Check sheet for the modelled part. Datum: model origin and axes. Units: mm. Give positions to 0.01 mm unless a question says otherwise; leave off trailing zeros. Loops run counter-clockwise (first coordinate to the right, second up) from the corner with the lowest first, then second, coordinate; pieces in that order, holes last.
```python
from build123d import *

# Parameters (mm, degrees)
SKETCH1_R           = 1.5
BOSS_EXTRUDE1_DEPTH = 3


with BuildPart() as part:
    # Sketch1 → Boss-Extrude1 (new body)
    with BuildSketch(Plane.XY):
        with BuildLine():
            Line((15.435057436, 20.921377099), (-0.10870117, 20.838196592))
            ThreePointArc((-0.10870117, 20.838196592), (-2.225289061, 19.948177695), (-3.092604315, 17.822185647))
            Line((-3.092604315, 17.822185647), (-2.998956565, 0.322436217))
            ThreePointArc((-2.998956565, 0.322436217), (-2.108937668, -1.794151674), (0.01705438, -2.661466928))
            Line((0.01705438, -2.661466928), (15.560812986, -2.578286421))
            ThreePointArc((15.560812986, -2.578286421), (17.766430895, -3.332819275), (19.891460268, -2.374528948))
            Line((19.891460268, -2.374528948), (30.659457178, -1.580311749))
            ThreePointArc((30.659457178, -1.580311749), (32.311987692, -0.938952483), (33.323696389, 0.516603879))
            ThreePointArc((33.323696389, 0.516603879), (33.38449749, 2.903690209), (32.146093551, 4.945315446))
            Line((32.146093551, 4.945315446), (32.099909063, 13.575709212))
            ThreePointArc((32.099909063, 13.575709212), (33.31639169, 15.630471471), (33.230046407, 18.016770366))
            ThreePointArc((33.230046407, 18.016770366), (32.202817639, 19.461415605), (30.543517656, 20.085052019))
            Line((30.543517656, 20.085052019), (19.767637393, 20.763979817))
            ThreePointArc((19.767637393, 20.763979817), (17.632473675, 21.699472247), (15.435057436, 20.921377099))
        make_face()
        with Locations((29.560164558, 17.392133017)):
            Circle(SKETCH1_R, mode=Mode.SUBTRACT)
        with Locations((29.65, 0.604781235)):
            Circle(SKETCH1_R, mode=Mode.SUBTRACT)
        with Locations((-0.101138608, 0.73794926)):
            Circle(SKETCH1_R, mode=Mode.SUBTRACT)
        with Locations((-0.190505318, 17.437710144)):
            Circle(SKETCH1_R, mode=Mode.SUBTRACT)
        Polygon((2.641027261, 11.552778262), (2.667248631, 6.652848422), (4.067228585, 6.660340242), (4.089168915, 2.560398947), (9.689088733, 2.590366227), (9.704072373, -0.209593682), (21.903897689, -0.144307821), (21.888914049, 2.655652087), (27.388835298, 2.685084237), (27.321944048, 15.184905259), (24.621982708, 15.170456748), (24.605393678, 18.270412362), (9.605608452, 18.190142862), (9.622197482, 15.090187248), (4.022277665, 15.060219968), (4.041007215, 11.560270082), align=None, mode=Mode.SUBTRACT)
    extrude(amount=BOSS_EXTRUDE1_DEPTH)


solid = part.part
```
(1) Release check for a two-part mould opening along Y. For faces 1 (the face through (32.22, 19.45, 1.48)), 2 (the face through (-1.3, 18.45, 1.48)), 3 (the face through (33.31, 15.6, 1.48)), 4 (the face through (17.733, -3.334, 1.479)) record: pulls with the +Y half, pulls with the -Y half, needs draft (parallel to the pull), parting line crosses it, or undercut.
(2) Section check D-D on z = 1.4. Give the number of separate pieces and of enclosed holes in the cut face, plus the area to 3 significant figures.
(3) Section check A-A on x = 17.5. Record the boundary of the cut face in (y, z), plus the area to 3 significant figures.
(4) Section check B-B on y = 9.75. Record the boundary of the cut face in (x, z).
(5) Material ranges on line 1 (X direction, y = 17, z = 1.45); line 2 (X direction, y = 0.25, z = 2.1); line 3 (Y direction, x = 29.65, z = 1.35), recorded low to high.
(6) Gauge pin test, flat ends, axial feed: pin 1 Ø2.5 at (x, y) = (-0.1, 0.74) entering from -Z; pin 2 Ø1 at (y, z) = (16.5, 1.5) entering from +X; pin 3 Ø1.5 at (x, z) = (19.5, 1.5) entering from -Y. Record the tip position at first contact, or that the pin passes through.
(7) Section check C-C on x = 29.65. Record the boundary of the cut face in (y, z), plus the area to 3 significant figures.
Computed values:
1. face 1: pulls with the +Y half
1. face 2: undercut
1. face 3: undercut
1. face 4: pulls with the -Y half
2. separate pieces: 1
2. enclosed holes: 5
2. area: 416 mm2
3. outline: (-3.33, 0) - (-0.17, 0) - (-0.17, 3) - (-3.33, 3) - close; (18.23, 0) - (21.7, 0) - (21.7, 3) - (18.23, 3) - close
3. area: 19.9 mm2
4. outline: (-3.05, 0) - (2.65, 0) - (2.65, 3) - (-3.05, 3) - close; (27.35, 0) - (32.12, 0) - (32.12, 3) - (27.35, 3) - close
5. line 1: x = -3.09 to -1.63, 1.24 to 9.61, 24.61 to 28.11, 31.01 to 33.44
5. line 2: x = -3 to -1.52, 1.32 to 9.7, 21.9 to 28.19, 31.11 to 33.22
5. line 3: y = -1.65 to -0.9, 2.1 to 15.89, 18.89 to 20.14
6. pin 1: passes through
6. pin 2: stops at x = 33.45
6. pin 3: stops at y = -3.13
7. outline: (-1.65, 0) - (-0.9, 0) - (-0.9, 3) - (-1.65, 3) - close; (2.1, 0) - (15.89, 0) - (15.89, 3) - (2.1, 3) - close; (18.89, 0) - (20.14, 0) - (20.14, 3) - (18.89, 3) - close
7. area: 47.4 mm2
